Autodesk Inventor part; units mm, degrees
ref_plane "XZ Plane" through (0, 0, 0) normal (0, 1, 0) x (-1, 0, 0)
ref_plane "XY Plane" through (0, 0, 0) normal (0, 0, 1) x (1, 0, 0)
sketch "Esquisse1" plane through (0, 0, 0) normal (0, 1, 0) x (-1, 0, 0)
  circle A0 centre (0, 0) radius 37.5
  line L0 (37.5, 0) -> (-37.5, 0)
  dimension "d0" = 75
revolve "Révolution1" add sketch "Esquisse1" angle 180 about axis through (-37.5, 0, 0) along (1, 0, 0) picked at (1.2379, -17.9235) contours A0 L0
sketch "Esquisse3" plane through (0, 0, 0) normal (0, -1, 0) x (1, 0, 0)
  circle A0 centre (0, 0) radius 37.5
extrude "Extrusion2" add sketch "Esquisse3" along normal blind 10
sketch "Esquisse4" plane through (0, -10, 0) normal (0, -1, 0) x (1, 0, 0)
  circle A0 centre (0, 0) radius 37.5
  line L0 (-52.5, 0) -> (52.5, 0)
  line L1 (34.3693, 15) -> (-34.3693, 15)
  line L2 (-34.3693, -15) -> (34.3693, -15)
  dimension "d8" = 15
  dimension "d9" = 15
extrude "Extrusion3" add sketch "Esquisse4" along normal blind 5 contours L0 A0 L1 | A0 L2 L0
ref_plane "Plan de construction1" through (25, 0, 0) normal (1, 0, 0) x (0, 1, 0)
sketch "Esquisse6" plane through (25, 0, 0) normal (1, 0, 0) x (0, 1, 0)
  line L0 (0, 37.5) -> (0, -37.5)
  circle A0 centre (21.2908, 16.8449) radius 7.533
  line L1 (27.3087, 12.3138) -> (15.2729, 21.376)
  line L2 (0, 0) -> (47.2705, 0) construction
ref_plane "Plan de construction2" through (34.3693, -10, 0) normal (0, 0, -1) x (-1, 0, 0)
revolve "Révolution2" add sketch "Esquisse6" angle 360 about axis through (25, 27.3087, 12.3138) along (0, -0.7988722, 0.6015008) picked at (22.6507, 18.9558) contours A0 L1
mirror "Symétrie1" about plane through (34.3693, -10, 0) normal (0, 0, -1) of "Révolution2"
sketch "Esquisse8" plane through (25, 0, 0) normal (1, 0, 0) x (0, 1, 0)
  line L0 (-10, -15) -> (-10, -15) construction
  line L1 (-10, -15) -> (-15, -15) construction
  line L2 (-15, 15) -> (-15, -15) construction
  line L3 (-10, 15) -> (-15, 15) construction
  line L4 (-10, 15) -> (-10, 15) construction
  line L5 (-10, 15) -> (-15, 15) construction
  line L6 (-15, -15) -> (-15, 15) construction
  line L7 (-10, -15) -> (-15, -15) construction
  line L8 (0, 37.5) -> (0, -37.5) construction
  line L9 (-15, 15) -> (-15, -15) construction
  line L10 (-15, 0) -> (31.9456, 0) construction
  line L11 (2.3018, 12.6924) -> (2.3018, -12.6924)
  line L12 (2.3018, -12.6924) -> (-5.9689, 0) construction
  line L13 (-5.9689, 0) -> (2.3018, 12.6924) construction
  spline S0 degree 2 poles (2.3018, -12.6924) (-5.9689, 0) (2.3018, 12.6924) knots 1 1 1 2 2 2
  line L14 (2.3018, 0) -> (-5.9689, 0) construction
  point P0 (0, 0)
extrude "Extrusion5" cut sketch "Esquisse8" along normal through all
equation "\"d9\" = d8"
properties part number "head3"
Can you work these out from the model? Positions are in its coordinate system, mm. A direction names the side the tool comes from. Coordinates: 2 decimals unless noted, no trailing zeros. Write each loop counter-clockwise with the first axis right and the second up, starting at its lowest first coordinate (ties: lowest second). Pieces come first, ordered by that corner, then holes. Notation, with made-up numbers: (75, -40) -> (125, -40) arc R26 cw to (125, -13) -> close; hole circle Ø5 at (59, 6). An arc over 180 degrees is marked (long way). Write each question's results on one line, items separated by ' | '. Start each with the question number.
Q1. Imagine slicing it at B-B (y = -6.5). Write out the boundary of the cut face in (x, z), then the cut area to 3 significant figures.
Q2. I'm going to push flat-ended pins straight in: pin 1 (1.5 mm diameter, centred on y = 26.5, z = 14.5, fed in from +X); pin 2 (8 mm diameter, centred on x = -16.5, y = 7, fed in from -Z); pin 3 (25 mm diameter, centred on x = -0.5, z = -31.5, fed in from -Y). Where does each tip first touch, or does it pass through?
Q3. Imagine slicing it at D-D (x = 23). Write out the boundary of the cut face in (y, z).
Q4. On a 3-axis mill with a long thin cutter (end or side, diameter ignored), from which of +Z, -Z, +X, -X, +Y, -Y can I reach the whole of each face in a straight line? I mean faces 4 (the face through (0, -12, -15)), 5 (the face through (0, -10, 24)), 6 (the face through (-1, -15, 0)). Say none if no direction works.
Q5. We'd pull the mould along Y, two halves only. Please class faces 1 (the face through (0, -12, 15)), 2 (the face through (31, 2.302, 0)), 3 (the face through (0, -10, -24)): +Y half, -Y half, draft (parallel to the pull), parting line (faces both ways), or undercut.
Q6. If I drill on probe 1 along Y at (x, z) = (25.5, 3.5); probe 2 along Z at (x, y) = (31, 22); probe 3 along Z at (x, y) = (20.5, 26), over which ranges is the centre line in solid material (lowest first)?
Q7. Imagine slicing it at A-A (x = 0). Write out the boundary of the cut face in (y, z).
Q8. Imagine slicing it at C-C (x = -10.5). Write out the boundary of the cut face in (y, z), then the cut area to 3 significant figures.
Taken from the geometry:
1) outline: circle Ø75 at (0, 0) | area: 4,420 mm^2
2) pin 1: stops at x = 30.67 | pin 2: stops at z = -34.82 | pin 3: stops at y = -10
3) outline: (-15, -15) -> (-10, -15) -> (-10, -29.62) -> (0, -29.62) arc R29.62 ccw to (18.16, -23.4) arc R7.26 ccw to (26.95, -12.29) arc R29.62 ccw to (26.95, 12.29) arc R7.26 ccw to (18.16, 23.4) arc R29.62 ccw to (0, 29.62) -> (-10, 29.62) -> (-10, 15) -> (-15, 15) -> close
4) face 4: -Z, +X, -X, -Y | face 5: +Z, +X, -X, -Y | face 6: +Z, -Z, +X, -X, -Y
5) face 1: draft | face 2: undercut | face 3: -Y half
6) probe 1: y = -15 to -1.52, 2.3 to 27.27 | probe 2: z = -21.34 to -12.35, 12.35 to 21.34 | probe 3: z = -20.63 to 20.63
7) outline: (-15, -15) -> (-10, -15) -> (-10, -37.5) -> (0, -37.5) arc R37.5 ccw to (0, 37.5) -> (-10, 37.5) -> (-10, 15) -> (-15, 15) -> close
8) outline: (-15, -15) -> (-10, -15) -> (-10, -36) -> (0, -36) arc R36 ccw to (0, 36) -> (-10, 36) -> (-10, 15) -> (-15, 15) -> close | area: 2,910 mm^2
